from build123d import *

# Parameters (mm, degrees)
SKETCH1_W                      = 60
SKETCH1_H                      = 297.5
BASE_FLANGE1_DEPTH             = 3
EDGE_FLANGE1_STRIP_W           = 14
EDGE_FLANGE1_STRIP_H           = 3
EDGE_FLANGE1_STRIP_CUT_DEPTH   = 297.5
EDGE_FLANGE1_DEPTH             = 297.5
EDGE_FLANGE2_STRIP_W           = 14
EDGE_FLANGE2_STRIP_H           = 3
EDGE_FLANGE2_STRIP_CUT_DEPTH   = 56
EDGE_FLANGE2_STRIP_2_W         = 14
EDGE_FLANGE2_STRIP_2_H         = 3
EDGE_FLANGE2_STRIP_CUT_2_DEPTH = 56
EDGE_FLANGE2_STRIP_3_W         = 14
EDGE_FLANGE2_STRIP_3_H         = 3
EDGE_FLANGE2_STRIP_CUT_3_DEPTH = 56
EDGE_FLANGE2_STRIP_4_W         = 14
EDGE_FLANGE2_STRIP_4_H         = 3
EDGE_FLANGE2_STRIP_CUT_4_DEPTH = 56
EDGE_FLANGE2_DEPTH             = 56
EDGE_FLANGE2_BEND_DEPTH        = 56
EDGE_FLANGE2_BEND_2_DEPTH      = 56
EDGE_FLANGE2_BEND_3_DEPTH      = 56
SKETCH18_R                     = 4.6
EXTRUDE1_DEPTH                 = 311.797763827


# Sheet-metal steps are written as plain solids
with BuildPart() as part:
    # Sketch1 → Base-Flange1 (new body)
    with BuildSketch(Plane(origin=(0, 0, 0), x_dir=(1, 0, 0), z_dir=(0, 1, 0))):
        Rectangle(SKETCH1_W, SKETCH1_H)
    extrude(amount=BASE_FLANGE1_DEPTH)

    # Edge-Flange1 strip (across the edge) → Edge-Flange1 strip cut (cut)
    with BuildSketch(Plane(origin=(-30, 3, -148.75), x_dir=(1, 0, 0), z_dir=(0, 0, 1))):
        with Locations((-3, -1.5)):
            Rectangle(EDGE_FLANGE1_STRIP_W, EDGE_FLANGE1_STRIP_H)
    extrude(amount=EDGE_FLANGE1_STRIP_CUT_DEPTH, mode=Mode.SUBTRACT)

    # Edge-Flange1 section (across the edge) → Edge-Flange1 (add)
    with BuildSketch(Plane(origin=(-30, 3, -148.75), x_dir=(1, 0, 0), z_dir=(0, 0, 1))):
        with BuildLine():
            Line((0, 1), (0, 57))
            Line((0, 57), (3, 57))
            Line((3, 57), (3, 1))
            ThreePointArc((3, 1), (3.292893219, 0.292893219), (4, 0))
            Line((4, 0), (4, -3))
            ThreePointArc((4, -3), (1.171572875, -1.828427125), (0, 1))
        make_face()
    extrude(amount=EDGE_FLANGE1_DEPTH)

    # Edge-Flange2 strip (across the edge) → Edge-Flange2 strip cut (cut)
    with BuildSketch(Plane(origin=(-30, 4, 148.75), x_dir=(0, 0, -1), z_dir=(0, 1, 0))):
        with Locations((-3, -1.5)):
            Rectangle(EDGE_FLANGE2_STRIP_W, EDGE_FLANGE2_STRIP_H)
    extrude(amount=EDGE_FLANGE2_STRIP_CUT_DEPTH, mode=Mode.SUBTRACT)

    # Edge-Flange2 strip 2 (across the edge) → Edge-Flange2 strip cut 2 (cut)
    with BuildSketch(Plane(origin=(30, 0, 148.75), x_dir=(0, 0, -1), z_dir=(-1, 0, 0))):
        with Locations((-3, -1.5)):
            Rectangle(EDGE_FLANGE2_STRIP_2_W, EDGE_FLANGE2_STRIP_2_H)
    extrude(amount=EDGE_FLANGE2_STRIP_CUT_2_DEPTH, mode=Mode.SUBTRACT)

    # Edge-Flange2 strip 3 (across the edge) → Edge-Flange2 strip cut 3 (cut)
    with BuildSketch(Plane(origin=(-30, 60, -148.75), x_dir=(0, 0, 1), z_dir=(0, -1, 0))):
        with Locations((-3, -1.5)):
            Rectangle(EDGE_FLANGE2_STRIP_3_W, EDGE_FLANGE2_STRIP_3_H)
    extrude(amount=EDGE_FLANGE2_STRIP_CUT_3_DEPTH, mode=Mode.SUBTRACT)

    # Edge-Flange2 strip 4 (across the edge) → Edge-Flange2 strip cut 4 (cut)
    with BuildSketch(Plane(origin=(-26, 0, -148.75), x_dir=(0, 0, 1), z_dir=(1, 0, 0))):
        with Locations((-3, -1.5)):
            Rectangle(EDGE_FLANGE2_STRIP_4_W, EDGE_FLANGE2_STRIP_4_H)
    extrude(amount=EDGE_FLANGE2_STRIP_CUT_4_DEPTH, mode=Mode.SUBTRACT)

    # Edge-Flange2 section (across the edge) → Edge-Flange2 (add)
    with BuildSketch(Plane(origin=(-30, 4, 148.75), x_dir=(0, 0, -1), z_dir=(0, 1, 0))):
        with BuildLine():
            Line((0, 1), (0, 37))
            Line((0, 37), (3, 37))
            Line((3, 37), (3, 1))
            ThreePointArc((3, 1), (3.292893219, 0.292893219), (4, 0))
            Line((4, 0), (4, -3))
            ThreePointArc((4, -3), (1.171572875, -1.828427125), (0, 1))
        make_face()
    extrude(amount=EDGE_FLANGE2_DEPTH)

    # Edge-Flange2 section 2 (across the edge) → Edge-Flange2 bend (add)
    with BuildSketch(Plane(origin=(30, 0, 148.75), x_dir=(0, 0, -1), z_dir=(-1, 0, 0))):
        with BuildLine():
            Line((0, 1), (0, 37))
            Line((0, 37), (3, 37))
            Line((3, 37), (3, 1))
            ThreePointArc((3, 1), (3.292893219, 0.292893219), (4, 0))
            Line((4, 0), (4, -3))
            ThreePointArc((4, -3), (1.171572875, -1.828427125), (0, 1))
        make_face()
    extrude(amount=EDGE_FLANGE2_BEND_DEPTH)

    # Edge-Flange2 section 3 (across the edge) → Edge-Flange2 bend 2 (add)
    with BuildSketch(Plane(origin=(-30, 60, -148.75), x_dir=(0, 0, 1), z_dir=(0, -1, 0))):
        with BuildLine():
            Line((0, 1), (0, 37))
            Line((0, 37), (3, 37))
            Line((3, 37), (3, 1))
            ThreePointArc((3, 1), (3.292893219, 0.292893219), (4, 0))
            Line((4, 0), (4, -3))
            ThreePointArc((4, -3), (1.171572875, -1.828427125), (0, 1))
        make_face()
    extrude(amount=EDGE_FLANGE2_BEND_2_DEPTH)

    # Edge-Flange2 section 4 (across the edge) → Edge-Flange2 bend 3 (add)
    with BuildSketch(Plane(origin=(-26, 0, -148.75), x_dir=(0, 0, 1), z_dir=(1, 0, 0))):
        with BuildLine():
            Line((0, 1), (0, 37))
            Line((0, 37), (3, 37))
            Line((3, 37), (3, 1))
            ThreePointArc((3, 1), (3.292893219, 0.292893219), (4, 0))
            Line((4, 0), (4, -3))
            ThreePointArc((4, -3), (1.171572875, -1.828427125), (0, 1))
        make_face()
    extrude(amount=EDGE_FLANGE2_BEND_3_DEPTH)

    # Sketch18 → Extrude1 (cut, through all)
    with BuildSketch(Plane.XY.offset(148.75)):
        with Locations((-47, 47.5)):
            Circle(SKETCH18_R)
        with Locations((-47, 17.5)):
            Circle(SKETCH18_R)
        with Locations((-12.5, -17)):
            Circle(SKETCH18_R)
        with Locations((17.5, -17)):
            Circle(SKETCH18_R)
    extrude(amount=-EXTRUDE1_DEPTH, mode=Mode.SUBTRACT)


solid = part.part
For this review, take the finished solid that the model builds, in its own axes (mm). A direction names the side the tool comes from. Give positions to 0.01 mm unless a question says otherwise; leave off trailing zeros. Write each loop counter-clockwise with the first axis right and the second up, starting at its lowest first coordinate (ties: lowest second). Pieces come first, ordered by that corner, then holes. Notation, with made-up numbers: (88, -30.5) -> (142, -30.5) arc R14 ccw to (142, -15.5) -> close; hole circle Ø6 at (57, 55.25). An arc over 180 degrees is marked (long way). Use CSV: the item, a comma, the result in double quotes.
Q1. Mouldability with a two-part tool opening along X and no side actions: class faces 4 (the face through (-44.877, 43.419, -147.229)), 5 (the face through (2, 0, -2)), 6 (the face through (-27, 32, -2)) as pulls with the +X half, pulls with the -X half, needs draft (parallel to the pull), parting line crosses it, or undercut.
Conclusion:
face 4,"undercut"
face 5,"needs draft"
face 6,"pulls with the +X half"
Q2. Take a section at D-D, the plane y = 17.5. Write out the cut boundary in (x, z).
Conclusion:
outline,"(-67, -148.75) -> (-51.6, -148.75) -> (-51.6, -145.75) -> (-67, -145.75) -> close; (-67, 145.75) -> (-51.6, 145.75) -> (-51.6, 148.75) -> (-67, 148.75) -> close; (-42.4, -148.75) -> (-31, -148.75) arc R4 ccw to (-27, -144.75) -> (-27, 144.75) arc R4 ccw to (-31, 148.75) -> (-42.4, 148.75) -> (-42.4, 145.75) -> (-31, 145.75) arc R1 cw to (-30, 144.75) -> (-30, -144.75) arc R1 cw to (-31, -145.75) -> (-42.4, -145.75) -> close"
Q3. Tool access review of faces 1 (the face through (-30, 32, -2)), 2 (the face through (2, -19, -145.75)), 3 (the face through (2, 3, -2)): name each direction out of +Z, -Z, +X, -X, +Y, -Y from which nothing blocks a thin tool from reaching the whole face with its end or side.
Conclusion:
face 1,"-X, +Y, -Y"
face 2,"+X, -X, -Y"
face 3,"+Z, -Z, +X, +Y"
Q4. To check wall thickness, follow probe 1 along Y at (x, z) = (-47, -147); probe 2 along Z at (x, y) = (15, -10.5); probe 3 along Y at (x, z) = (-24, 50.5). State the ranges of each line that lie inside material, in increasing order. Write a range as [from, to].
Conclusion:
probe 1,"[4, 12.9], [22.1, 42.9], [52.1, 60]"
probe 2,"[-148.75, -145.75], [145.75, 148.75]"
probe 3,"[0, 3]"
Q5. Take a section at B-B, the plane y = -4. Write out the cut boundary in (x, z).
Conclusion:
outline,"(-26, -148.75) -> (30, -148.75) -> (30, -145.75) -> (-26, -145.75) -> close; (-26, 145.75) -> (30, 145.75) -> (30, 148.75) -> (-26, 148.75) -> close"
Q6. Take a section at A-A, the plane x = -12.5. Write out the cut boundary in (y, z), then the cut area to 3 significant figures.
Conclusion:
outline,"(-37, -148.75) -> (-21.6, -148.75) -> (-21.6, -145.75) -> (-37, -145.75) -> close; (-37, 145.75) -> (-21.6, 145.75) -> (-21.6, 148.75) -> (-37, 148.75) -> close; (-12.4, -148.75) -> (-1, -148.75) arc R4 ccw to (3, -144.75) -> (3, 144.75) arc R4 ccw to (-1, 148.75) -> (-12.4, 148.75) -> (-12.4, 145.75) -> (-1, 145.75) arc R1 cw to (0, 144.75) -> (0, -144.75) arc R1 cw to (-1, -145.75) -> (-12.4, -145.75) -> close"
area,"1,050 mm2"
Q7. For P1, Ø7.5, axis at x = -47, y = 17.5, coming from the -Z side; P2, Ø10, axis at y = 32.5, z = -42, coming from the -X side; P3, Ø4.5, axis at y = -9.5, z = 147, coming from the -X side, all flat-tipped, find the tip position at first contact; note any pin that passes through.
Conclusion:
P1,"through"
P2,"x = -30"
P3,"x = -26"
Q8. Take a section at C-C, the plane x = -59.5. Write out the cut boundary in (y, z).
Conclusion:
outline,"(4, -148.75) -> (60, -148.75) -> (60, -145.75) -> (4, -145.75) -> close; (4, 145.75) -> (60, 145.75) -> (60, 148.75) -> (4, 148.75) -> close"
